from build123d import *

# Parameters (mm, degrees)
SKETCH1_R           = 0.75
BOSS_EXTRUDE1_DEPTH = 2
FILLET7_R           = 4
FILLET8_R           = 0.5
FILLET9_R           = 2
SKETCH2_R           = 1.5
CUT_EXTRUDE1_DEPTH  = 46.472229495
FILLET10_R          = 4
FILLET12_R          = 3


with BuildPart() as part:
    # Sketch1 → Boss-Extrude1 (new body)
    with BuildSketch(Plane.XY):
        with BuildLine():
            ThreePointArc((9.900055809, -1), (9.400055809, -0.5), (9.900055809, 0))
            Line((9.900055809, 0), (12.900055809, 0))
            Line((12.900055809, 0), (12.900055809, 12))
            Line((12.900055809, 12), (15.400055809, 14))
            Line((15.400055809, 14), (15.400055809, 15))
            Line((15.400055809, 15), (10.898257816, 15))
            ThreePointArc((10.898257816, 15), (10.399156812, 14.500898997), (9.900055809, 15))
            Line((9.900055809, 15), (9.900055809, 17))
            Line((9.900055809, 17), (1.900055809, 17))
            Line((1.900055809, 17), (1.900055809, 16))
            ThreePointArc((1.900055809, 16), (2.400055809, 15.5), (1.900055809, 15))
            Line((1.900055809, 15), (-0.099944191, 15))
            ThreePointArc((-0.099944191, 15), (-0.599944191, 14.5), (-1.099944191, 15))
            Line((-1.099944191, 15), (-1.099944191, 17))
            Line((-1.099944191, 17), (-21.109742569, 28.55266248))
            ThreePointArc((-21.109742569, 28.55266248), (-34.392766222, 13.978204373), (-32.979517798, -5.690457894))
            ThreePointArc((-32.979517798, -5.690457894), (-27.872628368, -7.772375219), (-22.467282567, -8.866421))
            ThreePointArc((-22.467282567, -8.866421), (-11.79863746, -9.716406126), (-1.099944191, -10))
            Line((-1.099944191, -10), (-1.099944191, -1))
            ThreePointArc((-1.099944191, -1), (-1.599944191, -0.5), (-1.099944191, 0))
            Line((-1.099944191, 0), (1.900055809, 0))
            ThreePointArc((1.900055809, 0), (2.400055809, -0.5), (1.900055809, -1))
            Line((1.900055809, -1), (1.900055809, -2))
            Line((1.900055809, -2), (9.900055809, -2))
            Line((9.900055809, -2), (9.900055809, -1))
        make_face()
        with Locations((-10.771610825, 5.790346428)):
            Circle(SKETCH1_R, mode=Mode.SUBTRACT)
    extrude(amount=BOSS_EXTRUDE1_DEPTH)

    # Fillet7
    fillet7_edges = [part.edges().sort_by_distance(p)[0] for p in [
        (-32.979517798, -5.690457894, 1),
        (-21.109742569, 28.55266248, 1),
    ]]
    fillet(fillet7_edges, radius=FILLET7_R)

    # Fillet8
    fillet8_edges = [part.edges().sort_by_distance(p)[0] for p in [
        (-1.099944191, 17, 1),
        (15.400055809, 15, 1),
        (15.400055809, 14, 1),
        (12.900055809, 0, 1),
        (-1.099944191, -10, 1),
    ]]
    fillet(fillet8_edges, radius=FILLET8_R)

    # Fillet9
    fillet9_edges = [part.edges().sort_by_distance(p)[0] for p in [
        (12.900055809, 12, 1),
    ]]
    fillet(fillet9_edges, radius=FILLET9_R)

    # Sketch2 → Cut-Extrude1 (cut, through all)
    with BuildSketch(Plane.XY.offset(2)):
        with Locations((-21.218823002, 25.151538482)):
            Circle(SKETCH2_R)
        with Locations((-31.071264961, -2.690457894)):
            Circle(SKETCH2_R)
        with BuildLine():
            Line((-18.019584713, 17.636691368), (-22.57366805, 18.711702598))
            ThreePointArc((-22.57366805, 18.711702598), (-27.700823696, 10.223376044), (-27.391868807, 0.311566946))
            ThreePointArc((-27.391868807, 0.311566946), (-18.997839896, -2.988434266), (-10.058124429, -4.184768964))
            ThreePointArc((-10.058124429, -4.184768964), (-8.812200112, -3.583264873), (-8.54147164, -2.226489037))
            ThreePointArc((-8.54147164, -2.226489037), (-9.58655744, -0.347195343), (-11.387108468, 0.828374779))
            ThreePointArc((-11.387108468, 0.828374779), (-15.771507704, 5.758234049), (-11.450792663, 10.744002859))
            Line((-11.450792663, 10.744002859), (-12.839873731, 14.232317382))
            Line((-12.839873731, 14.232317382), (-18.019584713, 17.636691368))
        make_face()
        with BuildLine():
            Line((-18.129721387, 22.502019429), (-4.273314926, 14.502019429))
            ThreePointArc((-4.273314926, 14.502019429), (-3.248795873, 14.776538482), (-3.523314926, 15.801057535))
            Line((-3.523314926, 15.801057535), (-17.379721387, 23.801057535))
            ThreePointArc((-17.379721387, 23.801057535), (-18.404240439, 23.526538482), (-18.129721387, 22.502019429))
        make_face()
    extrude(amount=-CUT_EXTRUDE1_DEPTH, mode=Mode.SUBTRACT)

    # Fillet10
    fillet10_edges = [part.edges().sort_by_distance(p)[0] for p in [
        (-27.391868807, 0.311566946, 1),
        (-22.57366805, 18.711702598, 1),
        (-18.019584713, 17.636691368, 1),
        (-12.839873731, 14.232317382, 1),
    ]]
    fillet(fillet10_edges, radius=FILLET10_R)

    # Fillet12
    fillet12_edges = [part.edges().sort_by_distance(p)[0] for p in [
        (-11.450792663, 10.744002859, 1),
    ]]
    fillet(fillet12_edges, radius=FILLET12_R)


solid = part.part
Check sheet for the modelled part. Datum: model origin and axes. Units: mm. A direction names the side the tool comes from. Round coordinates to 2 decimals unless told otherwise and drop trailing zeros. Loops run counter-clockwise (first coordinate to the right, second up) from the corner with the lowest first, then second, coordinate; pieces in that order, holes last. Notation, with made-up numbers: (57, 28) -> (101, 28) arc R11 ccw to (101, 49) -> close; hole circle Ø8 at (38, -11.75). An arc over 180 degrees is marked (long way). Put each result on its own line as item: value. Start each with the question number.
1. Section check A-A (x = -30.5). Enter the section's corners in (y, z).
2. Section check B-B (y = 4). Enter the section's corners in (x, z).
3. Section check C-C (x = 7). Enter the section's corners in (y, z), plus the area to 3 significant figures.
4. Gauge pin test, flat ends, axial feed: pin 1 (0.6 mm diameter, centred on x = 12, z = 0.5, fed in from +Y); pin 2 (8 mm diameter, centred on x = -0.5, y = 18.5, fed in from +Z); pin 3 (1.4 mm diameter, centred on x = -10.77, y = 5.79, fed in from -Z); pin 4 (0.5 mm diameter, centred on y = 16, z = 0.5, fed in from +X). Record the tip position at first contact, or that the pin passes through.
5. Scan lines: probe 1 along X at (y, z) = (17.5, 1.9); probe 2 along Y at (x, z) = (6, 0.9); probe 3 along X at (y, z) = (5.5, 0.75). Record each from-to range of solid material in increasing order.
6. Draft check along X on faces 1 (the face through (-15.636, 16.07, 1.014)), 2 (the face through (-11, 9, 2)), 3 (the face through (-34.45, 13.81, 0.99)). Enter one of: +X half, -X half, draft (parallel to the pull), parting line (faces both ways), or undercut.
7. Section check D-D (z = 0.85). Give the number of separate pieces and of enclosed holes in the cut face, plus the area to 3 significant figures.
8. Access from +Z, -Z, +X, -X, +Y, -Y to the whole of each face (thin tool, end or side, straight path). Record for faces 4 (the face through (9.9, 16, 1)), 5 (the face through (11, 0, 1)), 6 (the face through (0, 0, 1)), 7 (the face through (-11.3, 18.56, 1.01)).
Findings:
1. outline: (-6.84, 0) -> (-4.08, 0) -> (-4.08, 2) -> (-6.84, 2) -> close; (-1.3, 0) -> (21.15, 0) -> (21.15, 2) -> (-1.3, 2) -> close
2. outline: (-35.71, 0) -> (-28.18, 0) -> (-28.18, 2) -> (-35.71, 2) -> close; (-15.44, 0) -> (12.9, 0) -> (12.9, 2) -> (-15.44, 2) -> close
3. outline: (-2, 0) -> (17, 0) -> (17, 2) -> (-2, 2) -> close
3. area: 38.0 mm^2
4. pin 1: stops at y = 15
4. pin 2: stops at z = 2
4. pin 3: passes through
4. pin 4: stops at x = 9.9
5. probe 1: x = -32.86 to -23.65, -17.87 to -9.47, -6.47 to -1.97
5. probe 2: y = -2 to 17
5. probe 3: x = -35.77 to -28.27, -15.76 to -11.46, -10.08 to 12.9
6. face 1: undercut
6. face 2: draft
6. face 3: -X half
7. separate pieces: 1
7. enclosed holes: 5
7. area: 993 mm^2
8. face 4: +Z, -Z, +X, +Y
8. face 5: +Z, -Z, +X, -Y
8. face 6: +Z, -Z, -Y
8. face 7: +Z, -Z
